Input: part model. Units: mm. Frame: model coordinates. Face numbers are marked on the shaded views. A direction names the side the tool comes from. Coordinates: 2 decimals unless noted, no trailing zeros. Write each loop counter-clockwise with the first axis right and the second up, starting at its lowest first coordinate (ties: lowest second). Pieces come first, ordered by that corner, then holes. Notation, with made-up numbers: M -32.75,26 L 2.25,26 A26 cw 2.25,41 Z; hole C 52.25,17 d1. An arc over 180 degrees is marked long. Write each question's results on one line, items separated by ' | '. Start each with the question number.
1. Section query C-C, the plane y = -35. Output: boundary loops of the cut face in (x, z).
2. First-contact query: pin 1 (3.5 mm diameter, centred on x = 4.5, z = 17, fed in from +Y); pin 2 (3.5 mm diameter, centred on x = 5.5, z = -4, fed in from -Y); pin 3 (6 mm diameter, centred on x = 10.5, y = -26.5, fed in from +Z). Flat tips, straight axial feed; report the tip coordinate or a pass-through.
3. Pull-direction query (Z, two-part tool) for the marked faces 1, 2 and 3; classes: +Z half, -Z half, draft (parallel to the pull), parting line (faces both ways), or undercut.
4. Section query D-D, the plane x = 16.25. Output: boundary loops of the cut face in (y, z).
5. Ray query, probe 1 along Z at (x, y) = (2, -42); probe 2 along X at (y, z) = (-42.5, -3.5); probe 3 along Z at (x, y) = (11, -35). Return the intervals inside material, ascending.
6. Section query A-A, the plane z = 14.5. Output: boundary loops of the cut face in (x, y).
7. Set-up query: the marked faces 4, 5 and 6. Return all of +Z, -Z, +X, -X, +Y, -Y with unobstructed straight access to the full face (end or side cutting, diameter ignored); none if empty.
8. Section query B-B, the plane y = -42. Output: boundary loops of the cut face in (x, z), and give its area (3 significant figures).
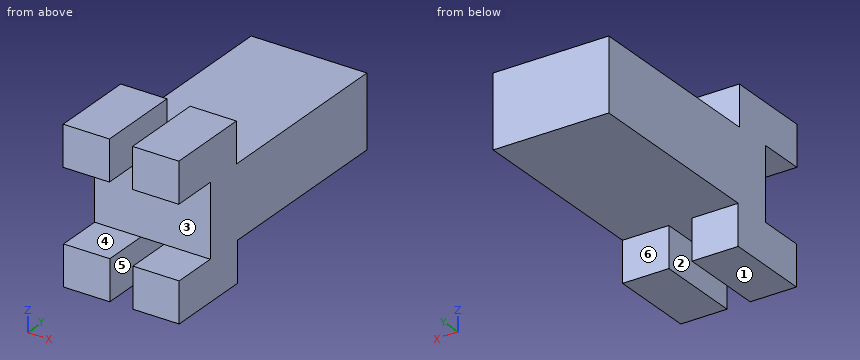
```python
from build123d import *

# Parameters (mm, degrees)
F0_W     = 20
F0_H     = 12.5
F1_DEPTH = 40
F2_W     = 8
F2_H     = 14.7096791708
F3_DEPTH = 7
F4_W     = 8
F4_H     = 7.9405596852
F4_H_2   = 6.9329673052
F5_DEPTH = 7


with BuildPart() as f1:
    # F0 (on Front) → F1 (new body)
    with BuildSketch(Plane.XZ):
        with Locations((10, 6.25)):
            Rectangle(F0_W, F0_H)
    extrude(amount=F1_DEPTH)

    # F2 (on face) → F3 (join)
    with BuildSketch(Plane.XY.offset(12.5)):
        with Locations((4, -40.6874705773)):
            Rectangle(F2_W, F2_H)
        with Locations((16, -40.6874705773)):
            Rectangle(F2_W, F2_H)
    extrude(amount=F3_DEPTH)

    # F4 (on face) → F5 (join)
    with BuildSketch(Plane(origin=(0, 0, 0), x_dir=(1, 0, 0), z_dir=(0, 0, -1))):
        with Locations((4, 43.9702798426)):
            Rectangle(F4_W, F4_H)
        with Locations((4, 36.5335163474)):
            Rectangle(F4_W, F4_H_2)
        with Locations((16, 36.5335163474)):
            Rectangle(F4_W, F4_H_2)
        with Locations((16, 43.9702798426)):
            Rectangle(F4_W, F4_H)
    extrude(amount=F5_DEPTH)


solid = f1.part
```
Answer:
1) outline: M 0,-7 L 8,-7 L 8,0 L 12,0 L 12,-7 L 20,-7 L 20,19.5 L 12,19.5 L 12,12.5 L 8,12.5 L 8,19.5 L 0,19.5 Z
2) pin 1: y = -33.33 | pin 2: y = -47.94 | pin 3: z = 12.5
3) face 1: -Z half | face 2: draft | face 3: undercut
4) outline: M -48.04,12.5 L -40,12.5 L -40,0 L -47.94,0 L -47.94,-7 L -33.07,-7 L -33.07,0 L 0,0 L 0,12.5 L -33.33,12.5 L -33.33,19.5 L -48.04,19.5 Z
5) probe 1: -7 to 0, 12.5 to 19.5 | probe 2: 0 to 8, 12 to 20 | probe 3: 0 to 12.5
6) outline: M 0,-48.04 L 8,-48.04 L 8,-33.33 L 0,-33.33 Z; M 12,-48.04 L 20,-48.04 L 20,-33.33 L 12,-33.33 Z
7) face 4: +X, -X, -Y | face 5: -Z, +Y, -Y | face 6: -Z, +X, -X, +Y
8) outline: M 0,-7 L 8,-7 L 8,0 L 0,0 Z; M 0,12.5 L 8,12.5 L 8,19.5 L 0,19.5 Z; M 12,-7 L 20,-7 L 20,0 L 12,0 Z; M 12,12.5 L 20,12.5 L 20,19.5 L 12,19.5 Z | area: 224 mm^2
